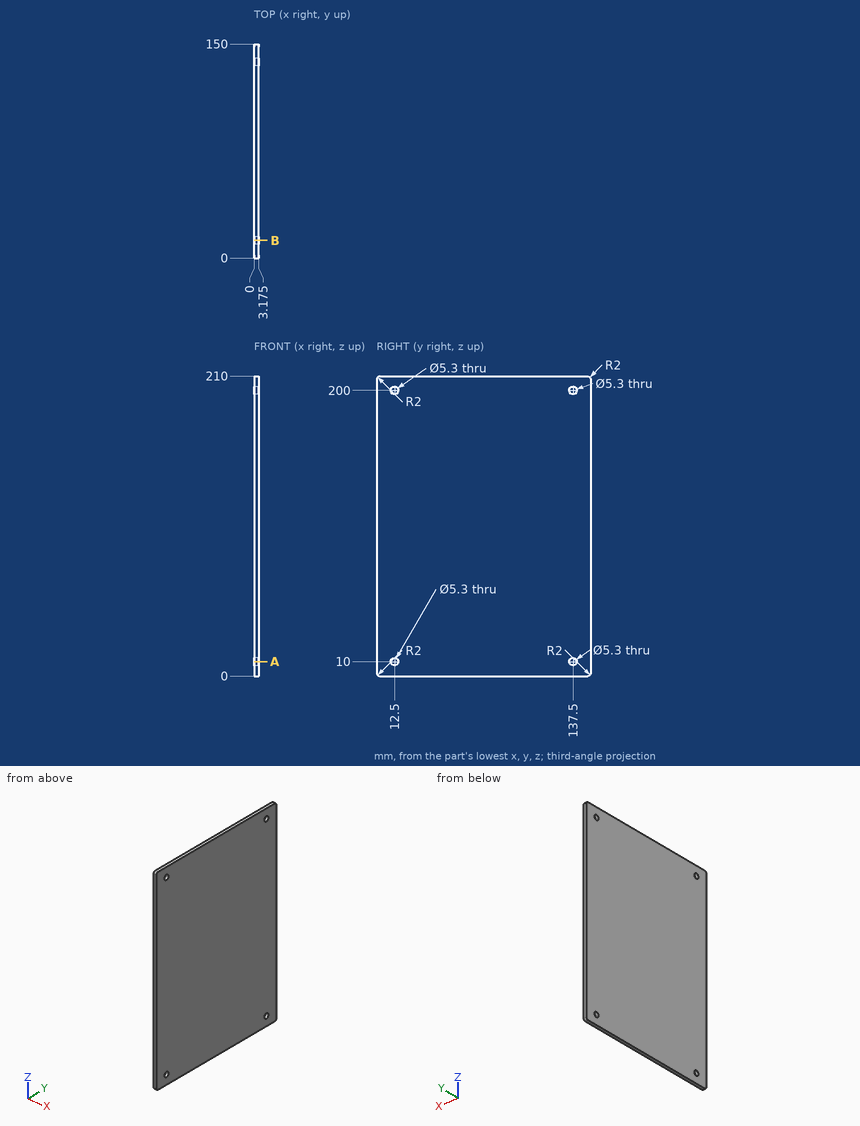
Answer from the drawing. Dimensions are ordinates in mm from the lowest x, y and z of the part. Coordinates: 2 decimals unless noted, no trailing zeros. Loops run counter-clockwise (first coordinate to the right, second up) from the corner with the lowest first, then second, coordinate; pieces in that order, holes last. Notation, with made-up numbers: (63, 54.25) - (88, 54.25) arc R13 ccw to (88, 77.25) - close; hole circle Ø6 at (18, -39). An arc over 180 degrees is marked (long way). Answer in a Markdown table with one row per item.
1. Given pin 1 (5 mm diameter, centred on y = 12.5, z = 200, fed in from -X), flat-ended and moving along its own axis, determine where the tip first touches the part or whether it passes through.
Conclusion:
| item | result |
|---|---|
| pin 1 | passes through |
2. Find section B-B, the plane y = 12.5. Write down the section's boundary in (x, z) (3 decimals).
Conclusion:
| item | result |
|---|---|
| outline | (0, 0) - (3.175, 0) - (3.175, 7.35) - (0, 7.35) - close; (0, 12.65) - (3.175, 12.65) - (3.175, 197.35) - (0, 197.35) - close; (0, 202.65) - (3.175, 202.65) - (3.175, 210) - (0, 210) - close |
3. Straight lines are drawn through the part: line 1 (Z direction, x = 1.65, y = 12); line 2 (Y direction, x = 2.45, z = 10); line 3 (Z direction, x = 1.55, y = 11). For each, find the intervals that lie inside material, in ascending order.
Conclusion:
| item | result |
|---|---|
| line 1 | z = 0 to 7.4, 12.6 to 197.4, 202.6 to 210 |
| line 2 | y = 0 to 9.85, 15.15 to 134.85, 140.15 to 150 |
| line 3 | z = 0 to 7.82, 12.18 to 197.82, 202.18 to 210 |
4. Find section A-A, the plane z = 10. Write down the section's boundary in (x, y) (3 decimals), then the cut area to 3 significant figures.
Conclusion:
| item | result |
|---|---|
| outline | (0, 0) - (3.175, 0) - (3.175, 9.85) - (0, 9.85) - close; (0, 15.15) - (3.175, 15.15) - (3.175, 134.85) - (0, 134.85) - close; (0, 140.15) - (3.175, 140.15) - (3.175, 150) - (0, 150) - close |
| area | 443 mm² |
